Could you check a few things on this model? Use its own coordinates, in mm. Give positions to 0.01 mm unless a question says otherwise; leave off trailing zeros. Loops run counter-clockwise (first coordinate to the right, second up) from the corner with the lowest first, then second, coordinate; pieces in that order, holes last. Notation, with made-up numbers: M 52,-34 L 64,-34 A21 ccw 64,-10 Z; hole C 13,78 d1. An arc over 180 degrees is marked long. Return JSON: item names as keys, results as strings. Group by question number.
1. If we section it at B-B (z = -29.5): Write out the boundary of the cut face in (x, y).
2. If we section it at A-A (x = -41): Write out the boundary of the cut face in (y, z), plus the area to 3 significant figures.
3. For pin 1 (5.5 mm diameter, centred on x = -6.24, z = -34.28, fed in from -Y); pin 2 (3 mm diameter, centred on y = 3.5, z = 37, fed in from -X); pin 3 (1.2 mm diameter, centred on x = 8, y = 2, fed in from +Z); pin 4 (1.8 mm diameter, centred on x = -43, y = 1.5, fed in from +Z), each with a flat end and sliding along its axis, tell me the tip position at first contact or that it passes through.
4. Please list where these lines run through material, in increasing order: line 1 (X direction, y = 4.9, z = 32.5); line 2 (X direction, y = 2.65, z = -29.5); line 3 (Z direction, x = -40, y = 3.55).
5. If we section it at D-D (x = 19.8): Write out the boundary of the cut face in (y, z).
6. If we section it at C-C (y = 1.7): Write out the boundary of the cut face in (x, z) (3 decimals), plus the area to 3 significant figures.
```python
from build123d import *

# Parameters (mm, degrees)
SKETCH1_W           = 35
SKETCH1_H           = 35
SKETCH1_W_2         = 50
SKETCH1_H_2         = 95
BOSS_EXTRUDE1_DEPTH = 6
FILLET1_R           = 10
SKETCH2_W           = 4
SKETCH2_H           = 20
CUT_EXTRUDE1_DEPTH  = 10
SKETCH3_W           = 40
SKETCH3_H           = 20
CUT_EXTRUDE2_DEPTH  = 7
SKETCH4_R           = 1.5
CUT_EXTRUDE3_DEPTH  = 7
SKETCH5_R           = 2.1
CUT_EXTRUDE4_DEPTH  = 7


with BuildPart() as part:
    # Sketch1 → Boss-Extrude1 (new body)
    with BuildSketch(Plane(origin=(0, 0, 0), x_dir=(1, 0, 0), z_dir=(0, 1, 0))):
        with Locations((-42.5, 30)):
            Rectangle(SKETCH1_W, SKETCH1_H)
        Rectangle(SKETCH1_W_2, SKETCH1_H_2)
    extrude(amount=BOSS_EXTRUDE1_DEPTH)

    # Fillet1
    fillet1_edges = [part.edges().sort_by_distance(p)[0] for p in [
        (-60, 3, -47.5),
        (-25, 3, -12.5),
        (-60, 3, -12.5),
    ]]
    fillet(fillet1_edges, radius=FILLET1_R)

    # Sketch2 → Cut-Extrude1 (cut)
    with BuildSketch(Plane(origin=(0, 6, 0), x_dir=(1, 0, 0), z_dir=(0, 1, 0))):
        with Locations((-7.36, -37.5)):
            Rectangle(SKETCH2_W, SKETCH2_H)
        with Locations((7.36, -37.5)):
            Rectangle(SKETCH2_W, SKETCH2_H)
    extrude(amount=-CUT_EXTRUDE1_DEPTH, mode=Mode.SUBTRACT)

    # Sketch3 → Cut-Extrude2 (cut, through all)
    with BuildSketch(Plane(origin=(0, 6, 0), x_dir=(1, 0, 0), z_dir=(0, 1, 0))):
        with Locations((-31, 29.5)):
            Rectangle(SKETCH3_W, SKETCH3_H)
    extrude(amount=-CUT_EXTRUDE2_DEPTH, mode=Mode.SUBTRACT)

    # Sketch4 → Cut-Extrude3 (cut, through all)
    with BuildSketch(Plane(origin=(0, 0, 0), x_dir=(-1, 0, 0), z_dir=(0, -1, 0))):
        with Locations((-19.8, 29.5)):
            Circle(SKETCH4_R)
    extrude(amount=-CUT_EXTRUDE3_DEPTH, mode=Mode.SUBTRACT)

    # Sketch5 → Cut-Extrude4 (cut, through all)
    with BuildSketch(Plane(origin=(0, 6, 0), x_dir=(1, 0, 0), z_dir=(0, 1, 0))):
        with Locations((-55.661145618, 24.425)):
            Circle(SKETCH5_R)
        with Locations((-55.661145618, 34.275)):
            Circle(SKETCH5_R)
        with Locations((-6.238854382, 34.275)):
            Circle(SKETCH5_R)
        with Locations((-6.238854382, 24.425)):
            Circle(SKETCH5_R)
    extrude(amount=-CUT_EXTRUDE4_DEPTH, mode=Mode.SUBTRACT)


solid = part.part
```
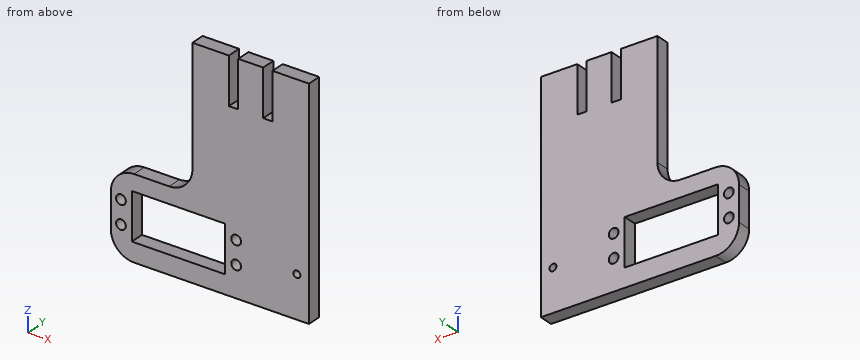
Answer:
{
 "1": {"outline": "M -60,0 L -51,0 L -51,6 L -60,6 Z; M -11,0 L 18.3,0 L 18.3,6 L -11,6 Z; M 21.3,0 L 25,0 L 25,6 L 21.3,6 Z"},
 "2": {"outline": "M 0,-47.5 L 6,-47.5 L 6,-39.5 L 0,-39.5 Z; M 0,-19.5 L 6,-19.5 L 6,-12.5 L 0,-12.5 Z", "area": "90.0 mm²"},
 "3": {"pin 1": "stops at y = 0", "pin 2": "stops at x = -25", "pin 3": "stops at z = 27.5", "pin 4": "stops at z = -12.5"},
 "4": {"line 1": "x = -25 to -9.36, -5.36 to 5.36, 9.36 to 25", "line 2": "x = -60 to -51, -11 to 18.3, 21.3 to 25", "line 3": "z = -47.5 to -39.5, -19.5 to -12.5"},
 "5": {"outline": "M 0,-47.5 L 6,-47.5 L 6,-31 L 0,-31 Z; M 0,-28 L 6,-28 L 6,47.5 L 0,47.5 Z"},
 "6": {"outline": "M -60,-37.5 A10 ccw -50,-47.5 L 25,-47.5 L 25,47.5 L 9.36,47.5 L 9.36,27.5 L 5.36,27.5 L 5.36,47.5 L -5.36,47.5 L -5.36,27.5 L -9.36,27.5 L -9.36,47.5 L -25,47.5 L -25,-2.5 A10 cw -35,-12.5 L -50,-12.5 A10 ccw -60,-22.5 Z; hole C -55.661,-34.275 d4.2; hole C -55.661,-24.425 d4.2; hole M -51,-39.5 L -11,-39.5 L -11,-19.5 L -51,-19.5 Z; hole C -6.239,-34.275 d4.2; hole C -6.239,-24.425 d4.2; hole C 19.8,-29.5 d3", "area": "4,930 mm²"}
}
